Source: CAD feature listing. Evaluate the final solid. Frame: model axes, mm. A direction names the side the tool comes from. Round coordinates to 2 decimals unless told otherwise and drop trailing zeros. Order: outer loops, then holes, each group sorted by start corner. A loop starts at its lowest first (then second) coordinate and runs counter-clockwise, first axis right, second up. Notation, with made-up numbers: (14.25, -30.75) - (22.25, -30.75) arc R22 cw to (22.25, -19.75) - close; hole circle Ø8 at (-29, 14). An arc over 180 degrees is marked (long way). Return JSON: item names as keys, results as strings. Group by question number.
1) Section D-D, the plane x = 69. Return loops of the section in (y, z).
2) Section C-C, the plane z = 22. Return loops of the section in (x, y).
3) Section B-B, the plane y = -7.5. Return loops of the section in (x, z), plus the area to 3 significant figures.
4) Access query for faces 1 (the cylindrical face through (12.325, -0.325, 40.536)), 2 (the flat face through (90, 0, 27)). Directions: +Z, -Z, +X, -X, +Y, -Y. A direction counts if a zero-diameter tool reaches every point of the face in a straight line with its end or side. Return the directions, or none.
5) Section A-A, the plane y = 0. Return loops of the section in (x, z).
6) Contact query for flat-ended pins moving along their axis: P1, Ø22.5, axis at x = 65, z = 55, coming from the +Y side; P2, Ø1.5, axis at y = 0.5, z = 22.5, coming from the -X side; P3, Ø5, axis at y = 8.5, z = 68, coming from the +X side. Output: stop coordinate, or through.
7) Mould query, pull axis Z, two halves, no side actions, for faces 3 (the flat face through (44, 0, 0)), 4 (the flat face through (44, 12.5, 41)), 5 (the cylindrical face through (12.325, -0.195, 23.487)), 6 (the flat face through (40, 0, 80)). Classes: pulls with the +Z half, pulls with the -Z half, needs draft (parallel to the pull), parting line crosses it, or undercut.
8) Ray query, line 1 (Z direction, x = 16, y = 0); line 2 (Z direction, x = 9, y = 0); line 3 (Z direction, x = 65, y = 7.25). Return the intervals inside material, ascending. Write a range as from..to.
```python
from build123d import *

# Parameters (mm, degrees)
F0_R     = 12.5
F1_DEPTH = 12.5
F2_DEPTH = 12.501
F3_DEPTH = 12.5
F4_R     = 1.5
F5_DEPTH = 25
F6_R     = 2.5
F7_DEPTH = 90.001


# Not quite as in the source:
# - a feature names something its author has since deleted; it is built from what else it names


with BuildPart() as f1:
    # F0 (on Front) → F1 (new body, symmetric)
    with BuildSketch(Plane.XZ):
        Polygon((25.6665702909, 80), (15.280091039, 80), (0, 60.2131655427), (0, 40.0504879653), align=None)
        with BuildLine():
            Line((65, 80), (25.6665702909, 80))
            Line((25.6665702909, 80), (0, 40.0504879653))
            Line((0, 40.0504879653), (0, 0))
            Line((0, 0), (90, 0))
            Line((90, 0), (90, 55))
            ThreePointArc((90, 55), (82.6776695297, 72.6776695297), (65, 80))
        make_face()
        with Locations((65, 55)):
            Circle(F0_R, mode=Mode.SUBTRACT)
    extrude(amount=F1_DEPTH, both=True)

    # F0 (on Front) → F2 (cut, through all)
    with BuildSketch(Plane.XZ):
        Polygon((25.6665702909, 80), (15.280091039, 80), (0, 60.2131655427), (0, 40.0504879653), align=None)
        with BuildLine():
            Line((65, 80), (25.6665702909, 80))
            Line((25.6665702909, 80), (0, 40.0504879653))
            Line((0, 40.0504879653), (0, 0))
            Line((0, 0), (90, 0))
            Line((90, 0), (90, 55))
            ThreePointArc((90, 55), (82.6776695297, 72.6776695297), (65, 80))
        make_face()
        with Locations((65, 55)):
            Circle(F0_R, mode=Mode.SUBTRACT)
    extrude(amount=-F2_DEPTH, mode=Mode.SUBTRACT)

    # F0 (on Front) → F3 (join, symmetric)
    with BuildSketch(Plane.XZ):
        Polygon((25.6665702909, 80), (15.280091039, 80), (0, 60.2131655427), (0, 40.0504879653), align=None)
        with BuildLine():
            Line((65, 80), (25.6665702909, 80))
            Line((25.6665702909, 80), (0, 40.0504879653))
            Line((0, 40.0504879653), (0, 0))
            Line((0, 0), (90, 0))
            Line((90, 0), (90, 55))
            ThreePointArc((90, 55), (82.6776695297, 72.6776695297), (65, 80))
        make_face()
        with Locations((65, 55)):
            Circle(F0_R, mode=Mode.SUBTRACT)
    extrude(amount=F3_DEPTH, both=True)

    # F4 (on Right) → F5 (cut)
    with BuildSketch(Plane.YZ):
        with Locations((0, 22)):
            Circle(F4_R)
        with Locations((0, 42)):
            Circle(F4_R)
    extrude(amount=F5_DEPTH, mode=Mode.SUBTRACT)

    # F6 (on face) → F7 (cut, through all)
    with BuildSketch(Plane.YZ.offset(90)):
        with Locations((0, 3.611382097)):
            Circle(F6_R)
    extrude(amount=-F7_DEPTH, mode=Mode.SUBTRACT)


solid = f1.part
```
Geometry check:
{
 "1": {"outline": "(-12.5, 0) - (12.5, 0) - (12.5, 43.16) - (-12.5, 43.16) - close; (-12.5, 66.84) - (12.5, 66.84) - (12.5, 79.68) - (-12.5, 79.68) - close; hole circle Ø5 at (0, 3.61)"},
 "2": {"outline": "(0, -12.5) - (90, -12.5) - (90, 12.5) - (0, 12.5) - (0, 1.5) - (25, 1.5) - (25, -1.5) - (0, -1.5) - close"},
 "3": {"outline": "(0, 0) - (90, 0) - (90, 55) arc R25 ccw to (65, 80) - (15.28, 80) - (0, 60.21) - close; hole circle Ø25 at (65, 55)", "area": "6,420 mm2"},
 "4": {"face 1": "-X", "face 2": "+Z, -Z, +X, +Y, -Y"},
 "5": {"outline": "(0, 0) - (90, 0) - (90, 1.11) - (0, 1.11) - close; (0, 6.11) - (90, 6.11) - (90, 55) arc R25 ccw to (65, 80) - (15.28, 80) - (0, 60.21) - (0, 43.5) - (25, 43.5) - (25, 40.5) - (0, 40.5) - (0, 23.5) - (25, 23.5) - (25, 20.5) - (0, 20.5) - close; hole circle Ø25 at (65, 55)"},
 "6": {"P1": "through", "P2": "x = 25", "P3": "x = 87.69"},
 "7": {"face 3": "pulls with the -Z half", "face 4": "needs draft", "face 5": "undercut", "face 6": "pulls with the +Z half"},
 "8": {"line 1": "0..1.11, 6.11..20.5, 23.5..40.5, 43.5..80", "line 2": "0..1.11, 6.11..20.5, 23.5..40.5, 43.5..71.87", "line 3": "0..42.5, 67.5..80"}
}
